Check sheet for the modelled part. Datum: model origin and axes. Units: mm. Face numbers are marked on the shaded views. A direction names the side the tool comes from. Give positions to 0.01 mm unless a question says otherwise; leave off trailing zeros. Write each loop counter-clockwise with the first axis right and the second up, starting at its lowest first coordinate (ties: lowest second). Pieces come first, ordered by that corner, then holes. Notation, with made-up numbers: M 41,7 L 83,7 A11 ccw 83,20 Z; hole C 41,23 d2. An arc over 180 degrees is marked long. One line per item, written item: value. Start each with the question number.
from build123d import *

# Parameters (mm, degrees)
F1_DEPTH    = 20
F3_DEPTH    = 10
F4_SIZE     = 3
F5_T1_DEPTH = 10.4919836734
F6_SIZE     = 5


# Not quite as in the source:
# - a fillet or chamfer that OpenCascade refuses, or shapes differently, is made with other operations: its cross-section is extruded or revolved along the edge and cut away or added


with BuildPart() as f1:
    # F0 (on Top) → F1 (new body)
    with BuildSketch(Plane.XY):
        Polygon((11, 17.275), (-14, 17.275), (-14, -17.275), (11, -17.275), (11, -10.275), (-7, -10.275), (-7, 10.275), (11, 10.275), align=None)
    extrude(amount=F1_DEPTH)

    # F2 (on face) → F3 (join)
    with BuildSketch(Plane.YZ.offset(11)):
        with BuildLine():
            ThreePointArc((22.275, 14), (19.625, 15.3124404748), (22.275, 16.6248809497))
            Line((22.275, 16.6248809497), (22.275, 20))
            Line((22.275, 20), (17.275, 20))
            Line((17.275, 20), (17.275, 0))
            Line((17.275, 0), (22.275, 0))
            Line((22.275, 0), (22.275, 3.3751190503))
            ThreePointArc((22.275, 3.3751190503), (19.625, 4.6875595252), (22.275, 6))
            Line((22.275, 6), (22.275, 14))
        make_face()
    extrude(amount=-F3_DEPTH)

    # F4
    f4_edges = [f1.edges().sort_by_distance(p)[0] for p in [
        (11, 10.275, 10),
        (11, -10.275, 10),
    ]]
    chamfer(f4_edges, length=F4_SIZE)

    # F5: chamfer of 0.1 on 4 edges, made by hand

    # F5_s2 → F5_t1 (cut)
    with BuildSketch(Plane.YZ.offset(0.7540081633)):
        with BuildLine():
            Line((22.2785318644, 16.7232142773), (22.1942442254, 16.6784020049))
            Line((22.1942442254, 16.6784020049), (22.193125709, 16.6767440179))
            ThreePointArc((22.193125709, 16.6767440179), (22.2348996139, 16.6520287441), (22.2737878788, 16.6232901127))
            Line((22.2737878788, 16.6232901127), (22.277, 16.6248809497))
            ThreePointArc((22.277, 16.6248809497), (22.277, 16.6740476135), (22.2805318644, 16.7232142773))
            Line((22.2805318644, 16.7232142773), (22.2785318644, 16.7232142773))
        make_face()
        with BuildLine():
            Line((22.1942442254, 13.9464789448), (22.2785318644, 13.9016666723))
            Line((22.2785318644, 13.9016666723), (22.2805318644, 13.9016666723))
            ThreePointArc((22.2805318644, 13.9016666723), (22.277, 13.9508333362), (22.277, 14))
            Line((22.277, 14), (22.2737878788, 14.0015908369))
            ThreePointArc((22.2737878788, 14.0015908369), (22.2348996139, 13.9728522055), (22.193125709, 13.9481369318))
            Line((22.193125709, 13.9481369318), (22.1942442254, 13.9464789448))
        make_face()
        with BuildLine():
            Line((22.2785318644, 6.0983333277), (22.1942442254, 6.0535210552))
            Line((22.1942442254, 6.0535210552), (22.193125709, 6.0518630682))
            ThreePointArc((22.193125709, 6.0518630682), (22.2348996139, 6.0271477945), (22.2737878788, 5.9984091631))
            Line((22.2737878788, 5.9984091631), (22.277, 6))
            ThreePointArc((22.277, 6), (22.277, 6.0491666638), (22.2805318644, 6.0983333277))
            Line((22.2805318644, 6.0983333277), (22.2785318644, 6.0983333277))
        make_face()
        with BuildLine():
            Line((22.2785318644, 3.2767857227), (22.1942442254, 3.3215979951))
            Line((22.1942442254, 3.3215979951), (22.193125709, 3.3232559821))
            ThreePointArc((22.193125709, 3.3232559821), (22.2348996139, 3.3479712559), (22.2737878788, 3.3767098873))
            Line((22.2737878788, 3.3767098873), (22.277, 3.3751190503))
            ThreePointArc((22.277, 3.3751190503), (22.277, 3.3259523865), (22.2805318644, 3.2767857227))
            Line((22.2805318644, 3.2767857227), (22.2785318644, 3.2767857227))
        make_face()
    extrude(amount=F5_T1_DEPTH, mode=Mode.SUBTRACT)

    # F6
    f6_edges = [f1.edges().sort_by_distance(p)[0] for p in [
        (-14, 17.275, 10),
        (-14, -17.275, 10),
    ]]
    chamfer(f6_edges, length=F6_SIZE)


solid = f1.part
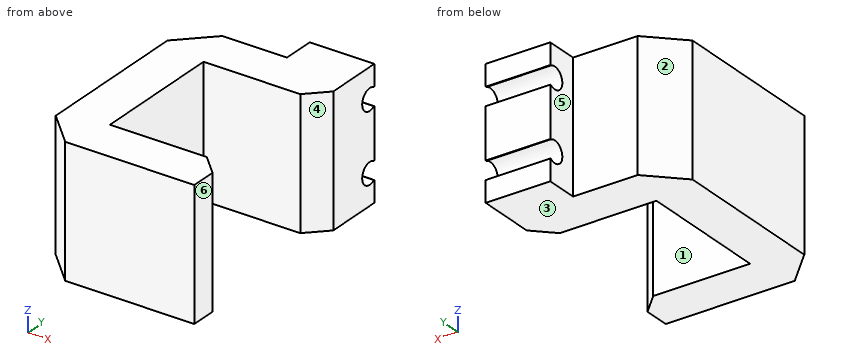
1) Cross-section at D-D (x = -8). Record the boundary of the cut face in (y, z) (3 decimals), plus the area to 3 significant figures.
2) Cross-section at A-A (x = 2). Record the boundary of the cut face in (y, z) (3 decimals), plus the area to 3 significant figures.
3) Tool access check on the marked faces 4, 5 and 6. Record the directions out of +Z, -Z, +X, -X, +Y, -Y that give a thin tool (end or side, any length) a straight path to the whole face; none if there is none.
4) Cross-section at C-C (y = 0). Record the boundary of the cut face in (x, z).
5) Draft check along Y on the marked faces 1, 2 and 3. Enter one of: released by +Y, released by -Y, zero draft, split by the parting line, or undercut.
6) Gauge pin test, flat ends, axial feed: pin 1 (4.5 mm diameter, centred on y = 21.28, z = 4.69, fed in from -X); pin 2 (8 mm diameter, centred on x = -5, z = 14, fed in from +Y) (3 decimals); pin 3 (2 mm diameter, centred on y = 4.5, z = 7, fed in from +X). Record the tip position at first contact, or that the pin passes through.
7) Cross-section at B-B (z = 8.5). Record the boundary of the cut face in (x, y) (3 decimals).
8) Material ranges on L1, parallel to Y at x = 3, z = 7.25 (3 decimals); L2, parallel to Y at x = 0, z = 6.5 (3 decimals); L3, parallel to X at y = 5, z = 2, recorded low to high. Write a range as from..to.
Data:
1. outline: M -17.275,0 L 17.275,0 L 17.275,20 L -17.275,20 Z
1. area: 691 mm2
2. outline: M -17.275,0 L -10.275,0 L -10.275,20 L -17.275,20 Z; M 10.275,0 L 22.275,0 L 22.275,3.279 L 22.198,3.32 A1.65 cw long 22.198,6.055 L 22.275,6.096 L 22.275,13.904 L 22.198,13.945 A1.65 cw long 22.198,16.68 L 22.275,16.721 L 22.275,20 L 10.275,20 Z
2. area: 365 mm2
3. face 4: +Z, -Z, +X
3. face 5: +Z, -Z, -X, +Y
3. face 6: +Z, -Z, +X, +Y, -Y
4. outline: M -14,0 L -7,0 L -7,20 L -14,20 Z
5. face 1: undercut
5. face 2: released by +Y
5. face 3: zero draft
6. pin 1: stops at x = 1
6. pin 2: stops at y = 17.275
6. pin 3: stops at x = -7
7. outline: M -14,-12.275 L -9,-17.275 L 11,-17.275 L 11,-13.275 L 8,-10.275 L -7,-10.275 L -7,10.275 L 8,10.275 L 11,13.275 L 11,22.275 L 1,22.275 L 1,17.275 L -9,17.275 L -14,12.275 Z
8. L1: y = -17.275..-10.275, 10.275..22.275
8. L2: y = -17.275..-10.275, 10.275..17.275
8. L3: x = -14..-7
